```python
from build123d import *

# Parameters (mm, degrees)
SKETCH_2_R          = 43
SKETCH_2_R_2        = 16.5
EXTRUDE_1_DEPTH     = 6
SKETCH_3_R          = 3
SKETCH_3_R_2        = 1.5
CUT_EXTRUDE_1_DEPTH = 6
CUT_EXTRUDE_5_DEPTH = 6
FILLET_2_R          = 3
SKETCH_6_R          = 43
SKETCH_6_R_2        = 42.9
CUT_EXTRUDE_6_DEPTH = 6
CUT_EXTRUDE_START   = -6
SKETCH_7_R          = 42.9
SKETCH_7_R_2        = 42.7
CUT_EXTRUDE_7_DEPTH = 6


with BuildPart() as part:
    # 草图2 → 凸台-拉伸1 (new body)
    with BuildSketch(Plane.XY):
        Circle(SKETCH_2_R)
        Circle(SKETCH_2_R_2, mode=Mode.SUBTRACT)
    extrude(amount=-EXTRUDE_1_DEPTH)

    # 草图3 → 切除-拉伸1 (cut)
    with BuildSketch(Plane.XY):
        with Locations((0, 29)):
            Circle(SKETCH_3_R)
        with Locations((29, 0)):
            Circle(SKETCH_3_R)
        with Locations((0, -29)):
            Circle(SKETCH_3_R)
        with Locations((-29, 0)):
            Circle(SKETCH_3_R)
        with Locations((-38.9, 0)):
            Circle(SKETCH_3_R_2)
        with Locations((0, 38.9)):
            Circle(SKETCH_3_R_2)
        with Locations((38.9, 0)):
            Circle(SKETCH_3_R_2)
        with Locations((0, -38.9)):
            Circle(SKETCH_3_R_2)
    extrude(amount=-CUT_EXTRUDE_1_DEPTH, mode=Mode.SUBTRACT)

    # 草图4 → 切除-拉伸5 (cut)
    with BuildSketch(Plane.XY):
        with BuildLine():
            ThreePointArc((-23.907618899, 7.309292618), (-17.67766953, 17.67766953), (-7.309292618, 23.907618899))
            Line((-7.309292618, 23.907618899), (-11.694868189, 38.252190239))
            ThreePointArc((-11.694868189, 38.252190239), (-28.284271247, 28.284271247), (-38.252190239, 11.694868189))
            Line((-38.252190239, 11.694868189), (-23.907618899, 7.309292618))
        make_face()
        with BuildLine():
            Line((11.694868189, 38.252190239), (7.309292618, 23.907618899))
            ThreePointArc((7.309292618, 23.907618899), (17.67766953, 17.67766953), (23.907618899, 7.309292618))
            Line((23.907618899, 7.309292618), (38.252190239, 11.694868189))
            ThreePointArc((38.252190239, 11.694868189), (28.284271247, 28.284271247), (11.694868189, 38.252190239))
        make_face()
        with BuildLine():
            Line((38.252190239, -11.694868189), (23.907618899, -7.309292618))
            ThreePointArc((23.907618899, -7.309292618), (17.67766953, -17.67766953), (7.309292618, -23.907618899))
            Line((7.309292618, -23.907618899), (11.694868189, -38.252190239))
            ThreePointArc((11.694868189, -38.252190239), (28.284271247, -28.284271247), (38.252190239, -11.694868189))
        make_face()
        with BuildLine():
            ThreePointArc((-7.309292618, -23.907618899), (-17.67766953, -17.67766953), (-23.907618899, -7.309292618))
            Line((-23.907618899, -7.309292618), (-38.252190239, -11.694868189))
            ThreePointArc((-38.252190239, -11.694868189), (-28.284271247, -28.284271247), (-11.694868189, -38.252190239))
            Line((-11.694868189, -38.252190239), (-7.309292618, -23.907618899))
        make_face()
    extrude(amount=-CUT_EXTRUDE_5_DEPTH, mode=Mode.SUBTRACT)

    # 圆角2
    fillet_2_edges = [part.edges().sort_by_distance(p)[0] for p in [
        (-38.252190239, -11.694868189, -3),
        (-23.907618899, -7.309292618, -3),
        (-7.309292618, -23.907618899, -3),
        (-11.694868189, -38.252190239, -3),
        (11.694868189, -38.252190239, -3),
        (7.309292618, -23.907618899, -3),
        (23.907618899, -7.309292618, -3),
        (38.252190239, -11.694868189, -3),
        (38.252190239, 11.694868189, -3),
        (23.907618899, 7.309292618, -3),
        (7.309292618, 23.907618899, -3),
        (11.694868189, 38.252190239, -3),
        (-11.694868189, 38.252190239, -3),
        (-7.309292618, 23.907618899, -3),
        (-23.907618899, 7.309292618, -3),
        (-38.252190239, 11.694868189, -3),
    ]]
    fillet(fillet_2_edges, radius=FILLET_2_R)

    # 草图6 → 切除-拉伸6 (cut)
    with BuildSketch(Plane.XY):
        Circle(SKETCH_6_R)
        Circle(SKETCH_6_R_2, mode=Mode.SUBTRACT)
    extrude(amount=-CUT_EXTRUDE_6_DEPTH, mode=Mode.SUBTRACT)

    # 草图7 → 切除-拉伸7 (cut)
    with BuildSketch(Plane(origin=(0, 0, -6), x_dir=(-1, 0, 0), z_dir=(0, 0, -1)).offset(CUT_EXTRUDE_START)):
        Circle(SKETCH_7_R)
        Circle(SKETCH_7_R_2, mode=Mode.SUBTRACT)
    extrude(amount=CUT_EXTRUDE_7_DEPTH, mode=Mode.SUBTRACT)


solid = part.part
```
Check sheet for the modelled part. Datum: model origin and axes. Units: mm. Coordinates: 2 decimals unless noted, no trailing zeros. Order: outer loops, then holes, each group sorted by start corner. A loop starts at its lowest first (then second) coordinate and runs counter-clockwise, first axis right, second up. Notation, with made-up numbers: (35.25, -32.75) -> (77.25, -32.75) arc R27 ccw to (77.25, -10.75) -> close; hole circle Ø4 at (67.25, 38). An arc over 180 degrees is marked (long way). Write each question's results on one line, items separated by ' | '. Start each with the question number.
1) Section check A-A (x = 0). Enter the section's corners in (y, z), and give its area (3 significant figures).
2) Section check D-D (y = 12). Enter the section's corners in (x, z), and give its area (3 significant figures).
3) Section check B-B (y = 34). Enter the section's corners in (x, z), and give its area (3 significant figures).
4) Depth check by flat-ended pin: pin 1 (1 mm diameter, centred on x = 28, z = -1.5, fed in from -Y). Enter the tip coordinate at first touch or a pass-through.
5) Material ranges on line 1 along Y through (x, z) = (0, -4.1); line 2 along Y through (x, z) = (-1, -0.45); line 3 along Y through (x, z) = (-29, -2.4), recorded low to high.
6) Section check C-C (x = 38.9). Enter the section's corners in (y, z), and give its area (3 significant figures).
7) Draft check along Y on faces 1 (the face through (-32, 0, -3)), 2 (the face through (-31.01, 9.48, -2.96)), 3 (the face through (9.257, -41.685, -2.958)). Enter one of: pulls with the +Y half, pulls with the -Y half, needs draft (parallel to the pull), parting line crosses it, or undercut.
Checked values:
1) outline: (-42.7, -6) -> (-40.4, -6) -> (-40.4, 0) -> (-42.7, 0) -> close; (-37.4, -6) -> (-32, -6) -> (-32, 0) -> (-37.4, 0) -> close; (-26, -6) -> (-16.5, -6) -> (-16.5, 0) -> (-26, 0) -> close; (16.5, -6) -> (26, -6) -> (26, 0) -> (16.5, 0) -> close; (32, -6) -> (37.4, -6) -> (37.4, 0) -> (32, 0) -> close; (40.4, -6) -> (42.7, -6) -> (42.7, 0) -> (40.4, 0) -> close | area: 206 mm²
2) outline: (-40.98, -6) -> (-36.89, -6) -> (-36.89, 0) -> (-40.98, 0) -> close; (-21.93, -6) -> (-11.32, -6) -> (-11.32, 0) -> (-21.93, 0) -> close; (11.32, -6) -> (21.93, -6) -> (21.93, 0) -> (11.32, 0) -> close; (36.89, -6) -> (40.98, -6) -> (40.98, 0) -> (36.89, 0) -> close | area: 176 mm²
3) outline: (-25.83, -6) -> (-21.07, -6) -> (-21.07, 0) -> (-25.83, 0) -> close; (-10.39, -6) -> (10.39, -6) -> (10.39, 0) -> (-10.39, 0) -> close; (21.07, -6) -> (25.83, -6) -> (25.83, 0) -> (21.07, 0) -> close | area: 182 mm²
4) pin 1: y = -32.67
5) line 1: -42.7 to -40.4, -37.4 to -32, -26 to -16.5, 16.5 to 26, 32 to 37.4, 40.4 to 42.7 | line 2: -42.69 to -40.02, -37.78 to -31.83, -26.17 to -16.47, 16.47 to 26.17, 31.83 to 37.78, 40.02 to 42.69 | line 3: -31.34 to -27.55, -8.87 to -3, 3 to 8.87, 27.55 to 31.34
6) outline: (-17.61, -6) -> (-1.5, -6) -> (-1.5, 0) -> (-17.61, 0) -> close; (1.5, -6) -> (17.61, -6) -> (17.61, 0) -> (1.5, 0) -> close | area: 193 mm²
7) face 1: undercut | face 2: undercut | face 3: parting line crosses it
